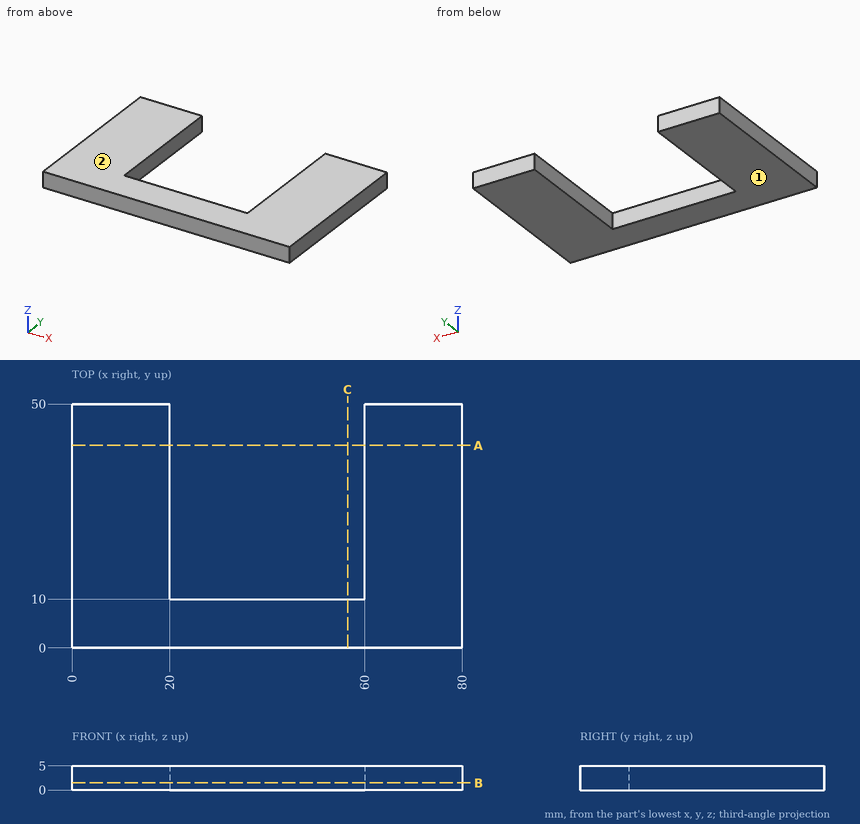
Answer from the drawing. Dimensions are ordinates in mm from the lowest x, y and z of the part. Coordinates: 2 decimals unless noted, no trailing zeros. Order: outer loops, then holes, each group sorted by start corner. A loop starts at its lowest first (then second) coordinate and runs counter-clockwise, first axis right, second up. Notation, with made-up numbers: M -32,70 L -8,70 A4 ccw -8,74 Z; hole C 8.5,-33.5 d1. An arc over 180 degrees is marked long. Put each result on its own line as item: value. Start each with the question number.
Item 1: The mould has two halves that part along Z. Classify the marked faces 1 and 2: +Z half, -Z half, draft (parallel to the pull), parting line (faces both ways), or undercut.
Item 2: Consider probe 1 along X at (y, z) = (36, 0.55); probe 2 along Y at (x, z) = (45, 3.8). Determine where each line is inside the solid, lowest interval first. Write a range as [from, to].
Item 3: Section B-B, the plane z = 1.5 is taken. Determine the outline of the cut face in (x, y).
Item 4: Section A-A, the plane y = 41.5 is taken. Determine the outline of the cut face in (x, z), plus the area to 3 significant figures.
Item 5: Section C-C, the plane x = 56.5 is taken. Determine the outline of the cut face in (y, z).
Computed:
1. face 1: -Z half
1. face 2: +Z half
2. probe 1: x = [0, 20], [60, 80]
2. probe 2: y = [0, 10]
3. outline: M 0,0 L 80,0 L 80,50 L 60,50 L 60,10 L 20,10 L 20,50 L 0,50 Z
4. outline: M 0,0 L 20,0 L 20,5 L 0,5 Z; M 60,0 L 80,0 L 80,5 L 60,5 Z
4. area: 200 mm2
5. outline: M 0,0 L 10,0 L 10,5 L 0,5 Z
